For this review, take the finished solid that the model builds, in its own axes (mm). Face numbers are marked on the shaded views. A direction names the side the tool comes from. Round coordinates to 2 decimals unless told otherwise and drop trailing zeros. Order: outer loops, then holes, each group sorted by start corner. A loop starts at its lowest first (then second) coordinate and runs counter-clockwise, first axis right, second up. Notation, with made-up numbers: M 59,55 L 113,55 A11 cw 113,72 Z; hole C 60,17 d8. An arc over 180 degrees is marked long. Use a Markdown table: item, result.
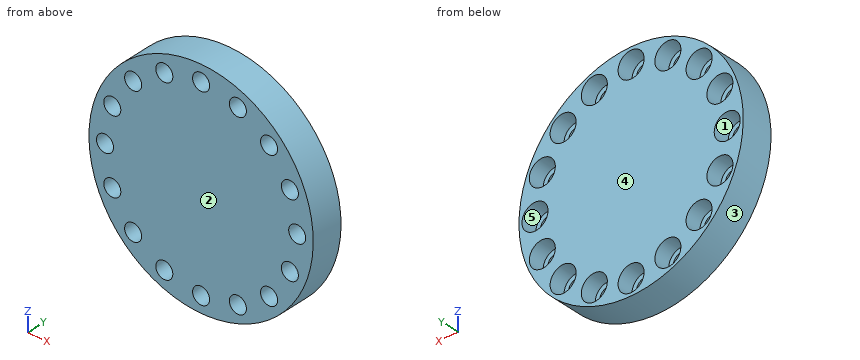
from build123d import *

# Parameters (mm, degrees)
SKETCH1_R                                        = 88.9
BOSS_EXTRUDE1_DEPTH                              = 25.4
CBORE_FOR_1_2_SOCKET_HEAD_CAP_SCREW1_D           = 13.49248
CBORE_FOR_1_2_SOCKET_HEAD_CAP_SCREW1_CBORE_D     = 20.6375
CBORE_FOR_1_2_SOCKET_HEAD_CAP_SCREW1_CBORE_DEPTH = 12.7
CIRPATTERN1_COUNT                                = 16


with BuildPart() as part:
    # Sketch1 → Boss-Extrude1 (new body)
    with BuildSketch(Plane(origin=(0, 0, 0), x_dir=(1, 0, 0), z_dir=(0, 1, 0))):
        with Locations(Location((0, 0, 0), (0, 0, 270))):
            Circle(SKETCH1_R)
    extrude(amount=-BOSS_EXTRUDE1_DEPTH)

    # CBORE for 1/2 Socket Head Cap Screw1 (through all)
    with Locations(Plane(origin=(0, 0, 0), x_dir=(1, 0, 0), z_dir=(0, 1, 0))):
        with Locations((0, 76.2)):
            cbore_for_1_2_socket_head_cap_screw1 = CounterBoreHole(CBORE_FOR_1_2_SOCKET_HEAD_CAP_SCREW1_D / 2, CBORE_FOR_1_2_SOCKET_HEAD_CAP_SCREW1_CBORE_D / 2, CBORE_FOR_1_2_SOCKET_HEAD_CAP_SCREW1_CBORE_DEPTH)

    # CirPattern1: CBORE for 1/2 Socket Head Cap Screw1 ×16 about axis
    cirpattern1_axis = Axis((0, 0, 0), (0, 1, 0))
    for i in range(1, CIRPATTERN1_COUNT):
        add(cbore_for_1_2_socket_head_cap_screw1.rotate(cirpattern1_axis, i * 360 / CIRPATTERN1_COUNT), mode=Mode.SUBTRACT)


solid = part.part
Q1. Wall thickness on line 1 along X through (y, z) = (-15.5, 0); line 2 along Z through (x, y) = (20, -9); line 3 along X through (y, z) = (-4.5, 77.5): over which ranges is each line inside the solid? List them lowest first. Write a range as [from, to].
Determined:
| item | result |
|---|---|
| line 1 | x = [-88.9, -82.95], [-69.45, 69.45], [82.95, 88.9] |
| line 2 | z = [-86.62, -75.15], [-65.65, 65.65], [75.15, 86.62] |
| line 3 | x = [-43.55, -36.65], [-21.67, -10.24], [10.24, 21.67], [36.65, 43.55] |
Q2. Add section C-C (y = -15.25). Give the number of separate pieces and of enclosed holes in the cut face, then the cut area to 3 significant figures.
Determined:
| item | result |
|---|---|
| separate pieces | 1 |
| enclosed holes | 16 |
| area | 22,500 mm^2 |
Q3. Add section A-A (z = 0). Write out the cut boundary in (x, y), then the cut area to 3 significant figures.
Determined:
| item | result |
|---|---|
| outline | M -88.9,-25.4 L -82.95,-25.4 L -82.95,-12.7 L -86.52,-12.7 L -86.52,0 L -88.9,0 Z; M -69.45,-25.4 L 69.45,-25.4 L 69.45,-12.7 L 65.88,-12.7 L 65.88,0 L -65.88,0 L -65.88,-12.7 L -69.45,-12.7 Z; M 82.95,-25.4 L 88.9,-25.4 L 88.9,0 L 86.52,0 L 86.52,-12.7 L 82.95,-12.7 Z |
| area | 3,650 mm^2 |
Q4. Add section B-B (x = 0). Write out the cut boundary in (y, z), then the cut area to 3 significant figures.
Determined:
| item | result |
|---|---|
| outline | M -25.4,-88.9 L 0,-88.9 L 0,-86.52 L -12.7,-86.52 L -12.7,-82.95 L -25.4,-82.95 Z; M -25.4,-69.45 L -12.7,-69.45 L -12.7,-65.88 L 0,-65.88 L 0,65.88 L -12.7,65.88 L -12.7,69.45 L -25.4,69.45 Z; M -25.4,82.95 L -12.7,82.95 L -12.7,86.52 L 0,86.52 L 0,88.9 L -25.4,88.9 Z |
| area | 3,650 mm^2 |
Q5. Draft analysis for pull direction Z (two halves, no side actions). For the marked faces 1, 2 and 3, state which applies: pulls with the +Z half, pulls with the -Z half, needs draft (parallel to the pull), parting line crosses it, or undercut.
Determined:
| item | result |
|---|---|
| face 1 | undercut |
| face 2 | needs draft |
| face 3 | parting line crosses it |
Q6. Machinability: for the marked faces 4 and 5, which of the approach directions +Z, -Z, +X, -X, +Y, -Y give a long, thin tool a straight path to every point of the face, cutting with its end or side? Answer none if there is none.
Determined:
| item | result |
|---|---|
| face 4 | +Z, -Z, +X, -X, +Y |
| face 5 | +Y |
Q7. Clearance check with flat-ended pins moving along their axes: pin 1 (8 mm diameter, centred on y = -15.5, z = -29.5, fed in from +X); pin 2 (10 mm diameter, centred on y = -16.5, z = 67.5, fed in from -X); pin 3 (8 mm diameter, centred on x = -13, z = 39, fed in from +Y); pin 4 (5 mm diameter, centred on y = -4.5, z = 69, fed in from +X). State where each tip first meets the part, or that it passes through.
Determined:
| item | result |
|---|---|
| pin 1 | stops at x = 85.16 |
| pin 2 | stops at x = -63.22 |
| pin 3 | stops at y = 0 |
| pin 4 | stops at x = 59 |
